```python
from build123d import *

# Parameters (mm, degrees)
SKETCH1_W               = 127
SKETCH1_H               = 101.6
BOSS_EXTRUDE1_DEPTH     = 12.7
CUT_EXTRUDE1_DEPTH      = 164.134453749
CUT_EXTRUDE1_DEPTH_BACK = 164.134453749
SKETCH2_R               = 2.4638
FILLET1_R               = 6.35


with BuildPart() as part:
    # Sketch1 → Boss-Extrude1 (new body)
    with BuildSketch(Plane(origin=(0, 0, 0), x_dir=(1, 0, 0), z_dir=(0, 1, 0))):
        with Locations((63.5, 50.8)):
            Rectangle(SKETCH1_W, SKETCH1_H)
    extrude(amount=BOSS_EXTRUDE1_DEPTH)

    # Sketch2 → Cut-Extrude1 (cut, two sides: drawn at the far end of the back side and taken through both)
    with BuildSketch(Plane(origin=(0, 12.7, 0), x_dir=(1, 0, 0), z_dir=(0, 1, 0)).offset(-CUT_EXTRUDE1_DEPTH_BACK)):
        with Locations(Location((31.75, 76.2, 0), (0, 0, 270))):
            Circle(SKETCH2_R)
        with Locations(Location((95.25, 76.2, 0), (0, 0, 270))):
            Circle(SKETCH2_R)
        with Locations(Location((95.25, 25.4, 0), (0, 0, 270))):
            Circle(SKETCH2_R)
        with Locations(Location((31.75, 25.4, 0), (0, 0, 270))):
            Circle(SKETCH2_R)
    extrude(amount=CUT_EXTRUDE1_DEPTH + CUT_EXTRUDE1_DEPTH_BACK, mode=Mode.SUBTRACT)

    # Fillet1
    fillet1_edges = [part.edges().sort_by_distance(p)[0] for p in [
        (0, 6.35, -101.6),
        (127, 6.35, -101.6),
        (127, 6.35, 0),
        (0, 6.35, 0),
    ]]
    fillet(fillet1_edges, radius=FILLET1_R)


solid = part.part
```
Check sheet for the modelled part. Datum: model origin and axes. Units: mm. Round coordinates to 2 decimals unless told otherwise and drop trailing zeros. Order: outer loops, then holes, each group sorted by start corner. A loop starts at its lowest first (then second) coordinate and runs counter-clockwise, first axis right, second up.
1) Mould release check, pull along Z, two halves, no side actions. Record for faces 1 (the cylindrical face through (1.81, 6.44, -99.69)), 2 (the cylindrical face through (34.193, 6.261, -25.721)), 3 (the flat face through (63, 6, 0)), 4 (the cylindrical face through (92.845, 6.261, -25.934)): +Z half, -Z half, draft (parallel to the pull), parting line (faces both ways), or undercut.
2) Scan lines: line 1 (X direction, y = 8.5, z = -25.4); line 2 (Z direction, x = 31.75, y = 3); line 3 (X direction, y = 7, z = -75). Record each from-to range of solid material in increasing order.
3) Section check B-B (x = 95.25). Record the boundary of the cut face in (y, z).
4) Section check A-A (z = -25.4). Record the boundary of the cut face in (x, y).
Result:
1. face 1: -Z half
1. face 2: undercut
1. face 3: +Z half
1. face 4: undercut
2. line 1: x = 0 to 29.29, 34.21 to 92.79, 97.71 to 127
2. line 2: z = -101.6 to -78.66, -73.74 to -27.86, -22.94 to 0
2. line 3: x = 0 to 29.6, 33.9 to 93.1, 97.4 to 127
3. outline: (0, -101.6) - (12.7, -101.6) - (12.7, -78.66) - (0, -78.66) - close; (0, -73.74) - (12.7, -73.74) - (12.7, -27.86) - (0, -27.86) - close; (0, -22.94) - (12.7, -22.94) - (12.7, 0) - (0, 0) - close
4. outline: (0, 0) - (29.29, 0) - (29.29, 12.7) - (0, 12.7) - close; (34.21, 0) - (92.79, 0) - (92.79, 12.7) - (34.21, 12.7) - close; (97.71, 0) - (127, 0) - (127, 12.7) - (97.71, 12.7) - close
